Verification items for the finished model (mm, model axes). Round coordinates to 2 decimals unless told otherwise and drop trailing zeros. Order: outer loops, then holes, each group sorted by start corner. A loop starts at its lowest first (then second) coordinate and runs counter-clockwise, first axis right, second up. Notation, with made-up numbers: M -26.75,30 L 23.25,30 A27 cw 23.25,55 Z; hole C 62.25,85.5 d10. An arc over 180 degrees is marked long. Return JSON: item names as keys, results as strings. Group by question number.
from build123d import *

# Parameters (mm, degrees)
SKETCH_1_W      = 90
SKETCH_1_H      = 14
SKETCH_1_R      = 1.5
SKETCH_1_W_2    = 70
SKETCH_1_H_2    = 8
EXTRUDE_1_DEPTH = 3
FILLET_1_R      = 3


with BuildPart() as part:
    # 草图1 → 凸台-拉伸1 (new body)
    with BuildSketch(Plane(origin=(0, 0, 0), x_dir=(1, 0, 0), z_dir=(0, 1, 0))):
        Rectangle(SKETCH_1_W, SKETCH_1_H)
        with Locations(Location((-40, 0, 0), (0, 0, 270))):
            Circle(SKETCH_1_R, mode=Mode.SUBTRACT)
        with Locations(Location((40, 0, 0), (0, 0, 90))):
            Circle(SKETCH_1_R, mode=Mode.SUBTRACT)
        Rectangle(SKETCH_1_W_2, SKETCH_1_H_2, mode=Mode.SUBTRACT)
    extrude(amount=EXTRUDE_1_DEPTH)

    # 圆角1
    fillet_1_edges = [part.edges().sort_by_distance(p)[0] for p in [
        (35, 1.5, 4),
        (35, 1.5, -4),
        (-35, 1.5, -4),
        (-35, 1.5, 4),
        (45, 1.5, 7),
        (-45, 1.5, 7),
        (-45, 1.5, -7),
        (45, 1.5, -7),
    ]]
    fillet(fillet_1_edges, radius=FILLET_1_R)


solid = part.part
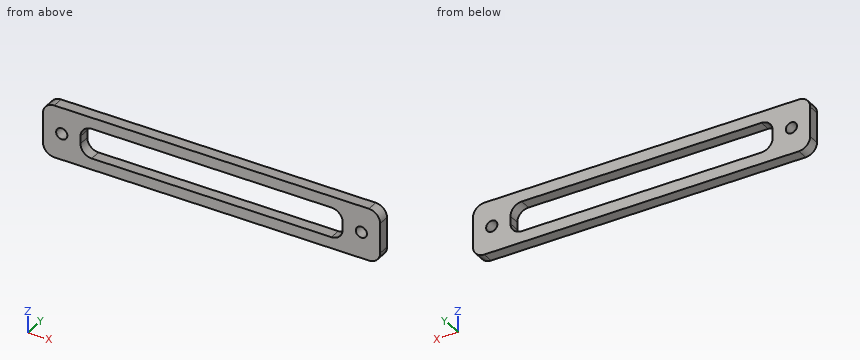
1. Cross-section at D-D (x = -40). Enter the section's corners in (y, z).
2. Go/stop test with a flat-tipped pin: pin 1 (3.5 mm diameter, centred on x = -40, z = 0, fed in from -Y). Record where the tip stops, or that it passes through.
3. Cross-section at B-B (z = 0). Enter the section's corners in (x, y).
4. Cross-section at A-A (x = 16). Enter the section's corners in (y, z), plus the area to 3 significant figures.
5. Cross-section at C-C (y = 0.6). Enter the section's corners in (x, z), plus the area to 3 significant figures.
6. Thickness scan on line 1 along X through (y, z) = (0.75, 0); line 2 along Z through (x, y) = (40, 2.4); line 3 along Z through (x, y) = (-15, 0.9). Record the ranges inside material, lowest first. Write a range as from..to.
Computed:
{
 "1": {"outline": "M 0,-7 L 3,-7 L 3,-1.5 L 0,-1.5 Z; M 0,1.5 L 3,1.5 L 3,7 L 0,7 Z"},
 "2": {"pin 1": "stops at y = 0"},
 "3": {"outline": "M -45,0 L -41.5,0 L -41.5,3 L -45,3 Z; M -38.5,0 L -35,0 L -35,3 L -38.5,3 Z; M 35,0 L 38.5,0 L 38.5,3 L 35,3 Z; M 41.5,0 L 45,0 L 45,3 L 41.5,3 Z"},
 "4": {"outline": "M 0,-7 L 3,-7 L 3,-4 L 0,-4 Z; M 0,4 L 3,4 L 3,7 L 0,7 Z", "area": "18.0 mm²"},
 "5": {"outline": "M -45,-4 A3 ccw -42,-7 L 42,-7 A3 ccw 45,-4 L 45,4 A3 ccw 42,7 L -42,7 A3 ccw -45,4 Z; hole C -40,0 d3; hole M -35,-1 A3 ccw -32,-4 L 32,-4 A3 ccw 35,-1 L 35,1 A3 ccw 32,4 L -32,4 A3 ccw -35,1 Z; hole C 40,0 d3", "area": "686 mm²"},
 "6": {"line 1": "x = -45..-41.5, -38.5..-35, 35..38.5, 41.5..45", "line 2": "z = -7..-1.5, 1.5..7", "line 3": "z = -7..-4, 4..7"}
}
